```python
from build123d import *

# Parameters (mm, degrees)
BOSS_EXTRUDE1_DEPTH = 3
SKETCH2_W           = 21
SKETCH2_H           = 40.6
CUT_EXTRUDE1_DEPTH  = 3


with BuildPart() as part:
    # Sketch1 → Boss-Extrude1 (new body)
    with BuildSketch(Plane.XY):
        Polygon((-38.890872965, 0), (0, 38.890872965), (38.890872965, 0), (0, -38.890872965), align=None)
    extrude(amount=BOSS_EXTRUDE1_DEPTH)

    # Sketch2 → Cut-Extrude1 (cut)
    with BuildSketch(Plane.XY.offset(3)):
        Rectangle(SKETCH2_W, SKETCH2_H)
    extrude(amount=-CUT_EXTRUDE1_DEPTH, mode=Mode.SUBTRACT)


solid = part.part
```
Could you check a few things on this model? Use its own coordinates, in mm. A direction names the side the tool comes from. Coordinates: 2 decimals unless noted, no trailing zeros. Write each loop counter-clockwise with the first axis right and the second up, starting at its lowest first coordinate (ties: lowest second). Pieces come first, ordered by that corner, then holes. Notation, with made-up numbers: (50.5, -39.75) -> (104.5, -39.75) arc R18 ccw to (104.5, -22.75) -> close; hole circle Ø1 at (64, -25). An arc over 180 degrees is marked (long way). Write item = value, one per line. Start each with the question number.
(1) Which directions (+Z, -Z, +X, -X, +Y, -Y) give clear straight access to the entire face, cutting with the end or side of a thin tool? Please do faces 5 (the face through (19.17, 19.72, 1.48)), 6 (the face through (10.5, 0, 2)).
(2) I want a section at C-C (z = 2.2). Please give me the cut outline in (x, y), plus the area to 3 significant figures.
(3) I want a section at D-D (y = 31.5). Please give me the cut outline in (x, z).
(4) I want a section at B-B (x = 7.5). Please give me the cut outline in (y, z).
(5) We'd pull the mould along X, two halves only. Please class faces 1 (the face through (-11, 0, 0)), 2 (the face through (0, -20.3, 2)), 3 (the face through (-19.17, -19.72, 1.48)), 4 (the face through (-10.5, 0, 2)): released by +X, released by -X, zero draft, split by the parting line, or undercut.
(6) Will these pins go through, and if not, where does the flat tip stop? pin 1 (1.5 mm diameter, centred on x = 0.5, z = 2, fed in from +Y); pin 2 (1.5 mm diameter, centred on x = -24.5, y = 16.5, fed in from -Z); pin 3 (0.9 mm diameter, centred on y = -2, z = 1, fed in from +X).
(7) I want a section at A-A (y = 12.5). Please give me the cut outline in (x, z).
(8) I need wall thicknesses on line 1 (Y direction, x = -7, z = 0.9); line 2 (X direction, y = 2.5, z = 0.3); line 3 (X direction, y = 3.5, z = 1.2). Which ranges of each line are inside material? Lowest first, please. Write a range as [from, to].
Result set:
q1.face_5 = +Z, -Z, +X, +Y
q1.face_6 = +Z, -Z
q2.outline = (-38.89, 0) -> (0, -38.89) -> (38.89, 0) -> (0, 38.89) -> close; hole (-10.5, -20.3) -> (10.5, -20.3) -> (10.5, 20.3) -> (-10.5, 20.3) -> close
q2.area = 2,170 mm2
q3.outline = (-7.39, 0) -> (7.39, 0) -> (7.39, 3) -> (-7.39, 3) -> close
q4.outline = (-31.39, 0) -> (-20.3, 0) -> (-20.3, 3) -> (-31.39, 3) -> close; (20.3, 0) -> (31.39, 0) -> (31.39, 3) -> (20.3, 3) -> close
q5.face_1 = zero draft
q5.face_2 = undercut
q5.face_3 = released by -X
q5.face_4 = undercut
q6.pin_1 = 38.89
q6.pin_2 = through
q6.pin_3 = 37.34
q7.outline = (-26.39, 0) -> (-10.5, 0) -> (-10.5, 3) -> (-26.39, 3) -> close; (10.5, 0) -> (26.39, 0) -> (26.39, 3) -> (10.5, 3) -> close
q8.line_1 = [-31.89, -20.3], [20.3, 31.89]
q8.line_2 = [-36.39, -10.5], [10.5, 36.39]
q8.line_3 = [-35.39, -10.5], [10.5, 35.39]
